Answer from the drawing. Dimensions are ordinates in mm from the lowest x, y and z of the part. Give positions to 0.01 mm unless a question says otherwise; leave off trailing zeros. Loops run counter-clockwise (first coordinate to the right, second up) from the corner with the lowest first, then second, coordinate; pieces in that order, holes last. Notation, with made-up numbers: M 67.5,29 L 126.5,29 A10 ccw 126.5,41 Z; hole C -39.75,21 d7. An arc over 180 degrees is marked long. Return JSON: item names as keys, results as strings. Group by question number.
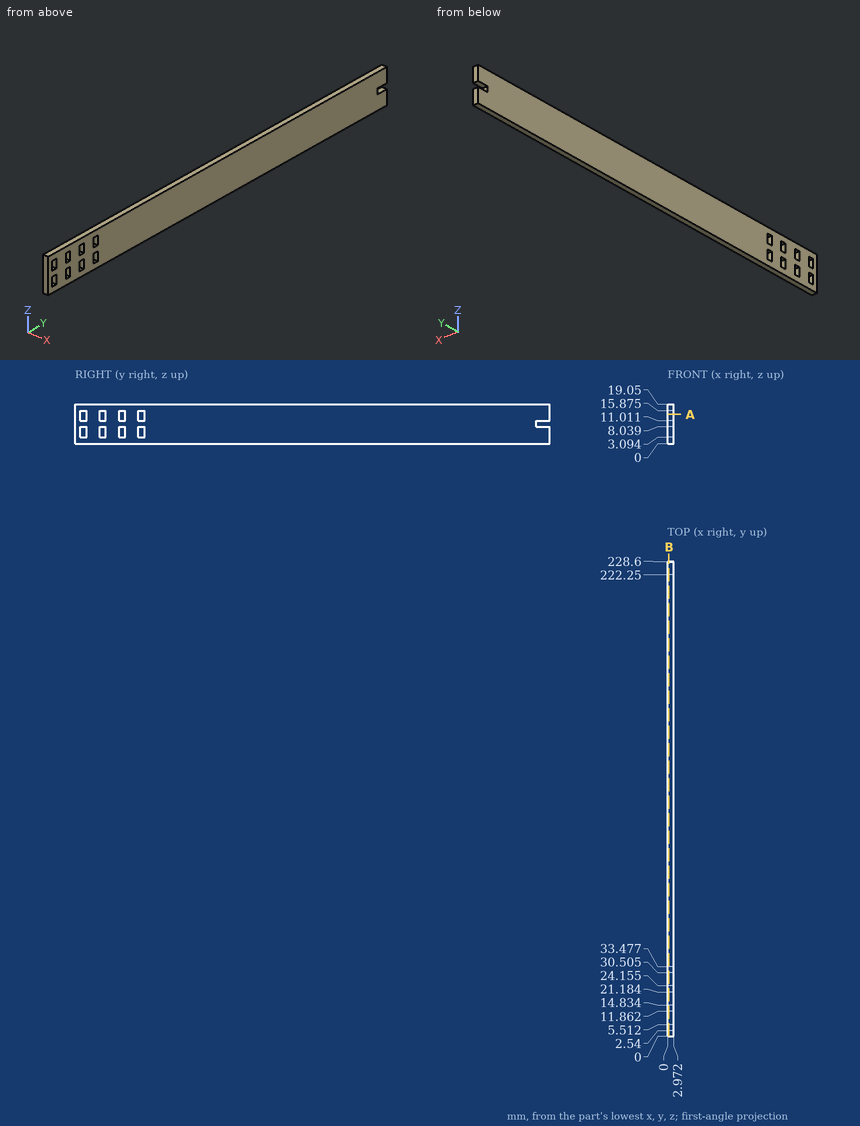
1. Straight lines are drawn through the part: line 1 along Y through (x, z) = (2.8, 15) (1 decimal); line 2 along Y through (x, z) = (1.15, 9.25). For each, find the intervals that lie inside material, in ascending order.
2. A flat-ended cylindrical pin translates along its axis: P1, Ø0.9, axis at x = 1.5, y = 22.5, coming from the -Z side. Find the tip coordinate at first contact, or state that the pin passes through.
3. Find section A-A (z = 14). Write down the section's boundary in (x, y) (1 decimal), and give its area (3 significant figures).
4. Find section B-B (x = 0.6). State how many separate pieces and enclosed holes the cut face has, and give its area (3 significant figures).
Result:
{
 "1": {"line 1": "y = 0 to 2.5, 5.5 to 11.9, 14.8 to 21.2, 24.2 to 30.5, 33.5 to 228.6", "line 2": "y = 0 to 222.25"},
 "2": {"P1": "stops at z = 0"},
 "3": {"outline": "M 0,0 L 3,0 L 3,2.5 L 0,2.5 Z; M 0,5.5 L 3,5.5 L 3,11.9 L 0,11.9 Z; M 0,14.8 L 3,14.8 L 3,21.2 L 0,21.2 Z; M 0,24.2 L 3,24.2 L 3,30.5 L 0,30.5 Z; M 0,33.5 L 3,33.5 L 3,228.6 L 0,228.6 Z", "area": "644 mm2"},
 "4": {"separate pieces": "1", "enclosed holes": "8", "area": "4,220 mm2"}
}
